```python
from build123d import *

# Parameters (mm, degrees)
SKETCH_1_R          = 1
EXTRUDE_1_DEPTH     = 1
CUT_EXTRUDE_START   = -1
SKETCH_2_W          = 14.5
SKETCH_2_H          = 2.048634766
SKETCH_2_W_2        = 15.468441373
CUT_EXTRUDE_1_DEPTH = 1


with BuildPart() as part:
    # 草图1 → 凸台-拉伸1 (new body)
    with BuildSketch(Plane(origin=(0, 0, 0), x_dir=(0, 0, -1), z_dir=(1, 0, 0))):
        with BuildLine():
            Line((35.439402333, 1.8), (35.439402333, 2.5))
            ThreePointArc((35.439402333, 2.5), (35.792955724, 3.353553391), (34.939402333, 3))
            Line((34.939402333, 3), (9.871490109, 3))
            ThreePointArc((9.871490109, 3), (9.017936719, 3.353553391), (9.371490109, 2.5))
            Line((9.371490109, 2.5), (9.371490109, 1.8))
            Line((9.371490109, 1.8), (4.371490109, 1.8))
            Line((4.371490109, 1.8), (4.371490109, 2.5))
            ThreePointArc((4.371490109, 2.5), (4.871240811, 2.984212798), (4.40304877, 3.499003057))
            Line((4.40304877, 3.499003057), (4.40304877, 4.175016197))
            Line((4.40304877, 4.175016197), (-7.761266908, 4.175016197))
            ThreePointArc((-7.761266908, 4.175016197), (-11.447420394, 3.667822703), (-10.564831187, 7.282516197))
            ThreePointArc((-10.564831187, 7.282516197), (-9.251899029, 7.163577788), (-8.295333824, 8.07072728))
            Line((-8.295333824, 8.07072728), (-7.691044908, 8.675016197))
            Line((-7.691044908, 8.675016197), (-8.295333824, 9.279305113))
            ThreePointArc((-8.295333824, 9.279305113), (-9.251899029, 10.186454606), (-10.564831187, 10.067516197))
            ThreePointArc((-10.564831187, 10.067516197), (-11.447420394, 13.682209691), (-7.761266908, 13.175016197))
            Line((-7.761266908, 13.175016197), (3.745661203, 13.175016197))
            ThreePointArc((3.745661203, 13.175016197), (3.988638874, 13.796186146), (4.40304877, 14.318828178))
            Line((4.40304877, 14.318828178), (4.40304877, 17.799978598))
            Line((4.40304877, 17.799978598), (4.40304877, 18.299978598))
            Line((4.40304877, 18.299978598), (4.40304877, 19.499978598))
            Line((4.40304877, 19.499978598), (4.40304877, 19.999978598))
            Line((4.40304877, 19.999978598), (9.90304877, 19.999978598))
            Line((9.90304877, 19.999978598), (10.40304877, 19.499978598))
            Line((10.40304877, 19.499978598), (17.439439899, 19.499978598))
            Line((17.439439899, 19.499978598), (18.9394023, 18.000016197))
            Line((18.9394023, 18.000016197), (21.9394023, 18.000016197))
            Line((21.9394023, 18.000016197), (24.9394023, 18.000016197))
            Line((24.9394023, 18.000016197), (26.439364701, 19.499978598))
            Line((26.439364701, 19.499978598), (34.439402333, 19.499978598))
            Line((34.439402333, 19.499978598), (34.939402333, 19.999978598))
            Line((34.939402333, 19.999978598), (40.439402333, 19.999978598))
            Line((40.439402333, 19.999978598), (40.439402333, 19.499978598))
            Line((40.439402333, 19.499978598), (40.439402333, 18.299978598))
            Line((40.439402333, 18.299978598), (40.439402333, 17.799978598))
            Line((40.439402333, 17.799978598), (40.439402333, 14.275016197))
            Line((40.439402333, 14.275016197), (40.439402333, 3.5))
            ThreePointArc((40.439402333, 3.5), (39.939402333, 3), (40.439402333, 2.5))
            Line((40.439402333, 2.5), (40.439402333, 1.8))
            Line((40.439402333, 1.8), (35.439402333, 1.8))
        make_face()
        with Locations((5.9394023, 12.675016197)):
            Circle(SKETCH_1_R, mode=Mode.SUBTRACT)
        with Locations((-9.776831345, 12.175016197)):
            Circle(SKETCH_1_R, mode=Mode.SUBTRACT)
        with Locations((-9.776831345, 5.175016197)):
            Circle(SKETCH_1_R, mode=Mode.SUBTRACT)
        with Locations((37.914877951, 12.675016197)):
            Circle(SKETCH_1_R, mode=Mode.SUBTRACT)
        with BuildLine():
            Line((19.3894023, 11.675016197), (19.3894023, 13.675016197))
            ThreePointArc((19.3894023, 13.675016197), (21.9394023, 16.225016197), (24.4894023, 13.675016197))
            Line((24.4894023, 13.675016197), (24.4894023, 11.675016197))
            ThreePointArc((24.4894023, 11.675016197), (21.9394023, 9.125016197), (19.3894023, 11.675016197))
        make_face(mode=Mode.SUBTRACT)
        with BuildLine():
            Line((27.369363454, 16.174920434), (27.369363454, 14.174920434))
            ThreePointArc((27.369363454, 14.174920434), (26.269363454, 13.074920434), (25.169363454, 14.174920434))
            Line((25.169363454, 14.174920434), (25.169363454, 16.174920434))
            ThreePointArc((25.169363454, 16.174920434), (26.269363454, 17.274920434), (27.369363454, 16.174920434))
        make_face(mode=Mode.SUBTRACT)
        with BuildLine():
            Line((16.510322262, 9.175620671), (16.510322262, 11.175620671))
            ThreePointArc((16.510322262, 11.175620671), (17.610322262, 12.275620671), (18.710322262, 11.175620671))
            Line((18.710322262, 11.175620671), (18.710322262, 9.175620671))
            ThreePointArc((18.710322262, 9.175620671), (17.610322262, 8.075620671), (16.510322262, 9.175620671))
        make_face(mode=Mode.SUBTRACT)
        with BuildLine():
            Line((27.368482338, 9.175620671), (27.368482338, 11.175620671))
            ThreePointArc((27.368482338, 11.175620671), (26.268482338, 12.275620671), (25.168482338, 11.175620671))
            Line((25.168482338, 11.175620671), (25.168482338, 9.175620671))
            ThreePointArc((25.168482338, 9.175620671), (26.268482338, 8.075620671), (27.368482338, 9.175620671))
        make_face(mode=Mode.SUBTRACT)
        with BuildLine():
            Line((16.509441146, 16.174920434), (16.509441146, 14.174920434))
            ThreePointArc((16.509441146, 14.174920434), (17.609441146, 13.074920434), (18.709441146, 14.174920434))
            Line((18.709441146, 14.174920434), (18.709441146, 16.174920434))
            ThreePointArc((18.709441146, 16.174920434), (17.609441146, 17.274920434), (16.509441146, 16.174920434))
        make_face(mode=Mode.SUBTRACT)
        with BuildLine():
            Line((10.40304877, 17.799978598), (10.40304877, 14.275016197))
            Line((10.40304877, 14.275016197), (14.101035123, 14.275016197))
            ThreePointArc((14.101035123, 14.275016197), (14.882875555, 16.44402539), (16.250834995, 18.299978598))
            Line((16.250834995, 18.299978598), (10.40304877, 18.299978598))
            Line((10.40304877, 18.299978598), (10.40304877, 17.799978598))
        make_face(mode=Mode.SUBTRACT)
        with BuildLine():
            Line((34.439402333, 17.799978598), (34.439402333, 14.275016197))
            Line((34.439402333, 14.275016197), (29.777769477, 14.275016197))
            ThreePointArc((29.777769477, 14.275016197), (28.995929045, 16.44402539), (27.627969606, 18.299978598))
            Line((27.627969606, 18.299978598), (34.439402333, 18.299978598))
            Line((34.439402333, 18.299978598), (34.439402333, 17.799978598))
        make_face(mode=Mode.SUBTRACT)
        with BuildLine():
            Line((36.439402333, 17.499978598), (38.439402333, 17.499978598))
            ThreePointArc((38.439402333, 17.499978598), (38.939402333, 16.999978598), (39.439402333, 17.499978598))
            Line((39.439402333, 17.499978598), (39.439402333, 18.499978598))
            ThreePointArc((39.439402333, 18.499978598), (38.939402333, 18.999978598), (38.439402333, 18.499978598))
            Line((38.439402333, 18.499978598), (36.439402333, 18.499978598))
            ThreePointArc((36.439402333, 18.499978598), (35.939402333, 18.999978598), (35.439402333, 18.499978598))
            Line((35.439402333, 18.499978598), (35.439402333, 17.499978598))
            ThreePointArc((35.439402333, 17.499978598), (35.939402333, 16.999978598), (36.439402333, 17.499978598))
        make_face(mode=Mode.SUBTRACT)
        with BuildLine():
            Line((6.40304877, 18.499978598), (8.40304877, 18.499978598))
            ThreePointArc((8.40304877, 18.499978598), (8.90304877, 18.999978598), (9.40304877, 18.499978598))
            Line((9.40304877, 18.499978598), (9.40304877, 17.499978598))
            ThreePointArc((9.40304877, 17.499978598), (8.90304877, 16.999978598), (8.40304877, 17.499978598))
            Line((8.40304877, 17.499978598), (6.40304877, 17.499978598))
            ThreePointArc((6.40304877, 17.499978598), (5.90304877, 16.999978598), (5.40304877, 17.499978598))
            Line((5.40304877, 17.499978598), (5.40304877, 18.499978598))
            ThreePointArc((5.40304877, 18.499978598), (5.90304877, 18.999978598), (6.40304877, 18.499978598))
        make_face(mode=Mode.SUBTRACT)
        with BuildLine():
            Line((3.923837863, 11.675016197), (-7.583090248, 11.675016197))
            ThreePointArc((-7.583090248, 11.675016197), (-7.611050301, 11.565186329), (-7.644505283, 11.456903696))
            Line((-7.644505283, 11.456903696), (-5.612617783, 9.425016197))
            Line((-5.612617783, 9.425016197), (4.40304877, 9.425016197))
            Line((4.40304877, 9.425016197), (4.40304877, 11.031204216))
            ThreePointArc((4.40304877, 11.031204216), (4.134505135, 11.331570544), (3.923837863, 11.675016197))
        make_face(mode=Mode.SUBTRACT)
        with BuildLine():
            Line((4.40304877, 5.675016197), (-7.583090248, 5.675016197))
            ThreePointArc((-7.583090248, 5.675016197), (-7.611050301, 5.784846064), (-7.644505283, 5.893128697))
            Line((-7.644505283, 5.893128697), (-5.612617783, 7.925016197))
            Line((-5.612617783, 7.925016197), (4.40304877, 7.925016197))
            Line((4.40304877, 7.925016197), (4.40304877, 5.675016197))
        make_face(mode=Mode.SUBTRACT)
    extrude(amount=EXTRUDE_1_DEPTH)

    # 草图2 → 切除-拉伸1 (cut)
    with BuildSketch(Plane(origin=(1, 0, 0), x_dir=(0, 0, -1), z_dir=(1, 0, 0)).offset(CUT_EXTRUDE_START)):
        with BuildLine():
            Line((13.939828478, 12.757591408), (9.40304877, 12.775016197))
            Line((9.40304877, 12.775016197), (8.18717898, 12.775016197))
            ThreePointArc((8.18717898, 12.775016197), (7.565363554, 11.119783095), (5.9394023, 10.425016197))
            Line((5.9394023, 10.425016197), (5.9394023, 7.637619031))
            Line((5.9394023, 7.637619031), (15.724530637, 7.637619031))
            ThreePointArc((15.724530637, 7.637619031), (14.385188615, 10.041794672), (13.939828478, 12.757591408))
        make_face()
        with BuildLine():
            Line((9.40304877, 15.823201902), (5.9394023, 15.823201902))
            Line((5.9394023, 15.823201902), (5.9394023, 14.925016197))
            ThreePointArc((5.9394023, 14.925016197), (6.794533869, 14.756181735), (7.521331502, 14.275016197))
            Line((7.521331502, 14.275016197), (9.40304877, 14.275016197))
            Line((9.40304877, 14.275016197), (9.40304877, 15.823201902))
        make_face()
        with Locations((13.1894023, 5.113301648)):
            Rectangle(SKETCH_2_W, SKETCH_2_H)
        with BuildLine():
            Line((38.907843673, 7.637619031), (38.907843673, 10.65597705))
            ThreePointArc((38.907843673, 10.65597705), (36.683529357, 10.791859103), (35.667101272, 12.775016197))
            Line((35.667101272, 12.775016197), (29.938777276, 12.775016197))
            ThreePointArc((29.938777276, 12.775016197), (29.4964794, 10.05002368), (28.154273964, 7.637619031))
            Line((28.154273964, 7.637619031), (38.907843673, 7.637619031))
        make_face()
        with Locations((31.173622986, 5.113301648)):
            Rectangle(SKETCH_2_W_2, SKETCH_2_H)
        with BuildLine():
            Line((38.907843673, 15.823201902), (35.439402333, 15.823201902))
            Line((35.439402333, 15.823201902), (35.439402333, 14.275016197))
            Line((35.439402333, 14.275016197), (36.332948749, 14.275016197))
            ThreePointArc((36.332948749, 14.275016197), (37.553466901, 14.895800304), (38.907843673, 14.694055343))
            Line((38.907843673, 14.694055343), (38.907843673, 15.823201902))
        make_face()
        with BuildLine():
            Line((19.9394023, 6.887619031), (23.9394023, 6.887619031))
            ThreePointArc((23.9394023, 6.887619031), (24.6894023, 7.637619031), (23.9394023, 8.387619031))
            Line((23.9394023, 8.387619031), (19.9394023, 8.387619031))
            ThreePointArc((19.9394023, 8.387619031), (19.1894023, 7.637619031), (19.9394023, 6.887619031))
        make_face()
    extrude(amount=CUT_EXTRUDE_1_DEPTH, mode=Mode.SUBTRACT)


solid = part.part
```
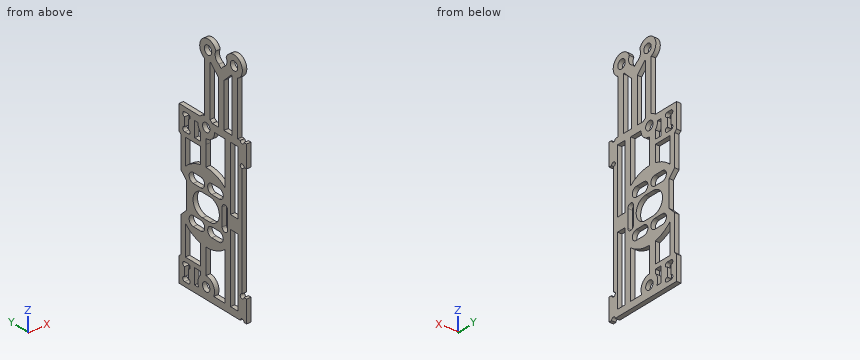
CAD build for the part. Positions are in the model's coordinates, mm. Coordinates: 2 decimals unless noted, no trailing zeros. Loops run counter-clockwise (first coordinate to the right, second up) from the corner with the lowest first, then second, coordinate; pieces in that order, holes last. Notation, with made-up numbers: (-28, 86.25) - (7, 86.25) arc R18 ccw to (7, 99.25) - close; hole circle Ø4 at (54.5, 88.5). An arc over 180 degrees is marked (long way). Return JSON: item names as keys, results as strings.
1. Band-saw the part on A-A (z = -22.5). Give the cut face in (x, y).
Result:
{"outline": "(0, 3) - (1, 3) - (1, 6.89) - (0, 6.89) - close; (0, 8.39) - (1, 8.39) - (1, 9.19) - (0, 9.19) - close; (0, 16.16) - (1, 16.16) - (1, 18) - (0, 18) - close"}
2. Band-saw the part on C-C (x = 0.65). State how many separate pieces and enclosed holes the cut face has, and give its area (3 significant figures).
Result:
{"separate pieces": "1", "enclosed holes": "22", "area": "405 mm2"}
3. Drop flat-ended pins along their axis: pin 1 (1.5 mm diameter, centred on y = 8.5, z = -13, fed in from +X); pin 2 (0.5 mm diameter, centred on x = 0.5, z = -31, fed in from +Y). Give the stop position or say it passes through.
Result:
{"pin 1": "passes through", "pin 2": "stops at y = 19.5"}
4. Probe L1, parallel to Y at x = 0.3, z = -30.5; L2, parallel to Y at x = 0.9, z = -2.5; L3, parallel to Z at x = 0.7, y = 5.25. List the from-to ranges inside material, lowest first. Write a range as from..to.
Result:
{"L1": "y = 3..4.09, 6.14..7.64, 12.78..14.28, 18.3..19.5", "L2": "y = 4.18..5.68, 7.93..9.43, 11.68..13.18", "L3": "z = -40.44..-38.91, -23.44..-20.44, -5.94..8.78, 10.77..12.03"}
5. Band-saw the part on B-B (z = 9.5). Give the cut face in (x, y).
Result:
{"outline": "(0, 2.94) - (1, 2.94) - (1, 4.21) - (0, 4.21) - close; (0, 6.14) - (1, 6.14) - (1, 7.1) - (0, 7.1) - close; (0, 10.25) - (1, 10.25) - (1, 11.21) - (0, 11.21) - close; (0, 13.14) - (1, 13.14) - (1, 14.41) - (0, 14.41) - close"}
